```python
from build123d import *

# Parameters (mm, degrees)
SKETCH1_W           = 2
SKETCH1_H           = 6
BOSS_EXTRUDE1_DEPTH = 3


with BuildPart() as part:
    # Sketch1 → Boss-Extrude1 (new body)
    with BuildSketch(Plane(origin=(0, 0, 0), x_dir=(1, 0, 0), z_dir=(0, 1, 0))):
        Polygon((0, 6), (0, 0), (40, 0), (40, 6), (40, 19), (40, 25), (33, 25), (33, 13), (20, 13), (7, 13), (7, 25), (0, 25), (0, 19), align=None)
        with Locations((-1, 22)):
            Rectangle(SKETCH1_W, SKETCH1_H)
        with Locations((-1, 3)):
            Rectangle(SKETCH1_W, SKETCH1_H)
        with Locations((41, 3)):
            Rectangle(SKETCH1_W, SKETCH1_H)
        with Locations((41, 22)):
            Rectangle(SKETCH1_W, SKETCH1_H)
    extrude(amount=BOSS_EXTRUDE1_DEPTH)


solid = part.part
```
Can you work these out from the model? Positions are in its coordinate system, mm. A direction names the side the tool comes from. Coordinates: 2 decimals unless noted, no trailing zeros. Loops run counter-clockwise (first coordinate to the right, second up) from the corner with the lowest first, then second, coordinate; pieces in that order, holes last. Notation, with made-up numbers: M 64,36.25 L 98,36.25 A19 cw 98,65.25 Z; hole C -12.5,78.5 d4. An arc over 180 degrees is marked long. Put each result on its own line as item: value. Start each with the question number.
(1) Imagine slicing it at C-C on x = 25. List the corners of the cut face in (y, z) for me.
(2) Which directions (+Z, -Z, +X, -X, +Y, -Y) give clear straight access to the entire face, cutting with the end or side of a thin tool? Please do faces 1 (the face through (-1, 1, -19)), 2 (the face through (3, 1, -25)), 3 (the face through (40, 1, -12)), 4 (the face through (7, 1, -19)).
(3) Imagine slicing it at B-B on y = 0.7. List the corners of the cut face in (x, z) for me.
(4) Imagine slicing it at A-A on z = -15. List the corners of the cut face in (x, y) for me, and give its area (3 significant figures).
(5) We'd pull the mould along Z, two halves only. Please class faces 5 (the face through (41, 1, -6)), 6 (the face through (20, 1, -13)), 7 (the face through (42, 1, -3)): +Z half, -Z half, draft (parallel to the pull), parting line (faces both ways), or undercut.
(6) Will these pins go through, and if not, where does the flat tip stop? pin 1 Ø1 at (x, y) = (13, 2.5) entering from -Z; pin 2 Ø5 at (x, z) = (3.5, -8.5) entering from -Y; pin 3 Ø10 at (x, z) = (12.5, -19.5) entering from +Y; pin 4 Ø0.9 at (y, z) = (1.5, -11.5) entering from -X.
(7) I need wall thicknesses on probe 1 along X at (y, z) = (2.45, -20.5); probe 2 along X at (y, z) = (1.1, -18.25); probe 3 along Z at (x, y) = (11, 2.2). Which ranges of each line are inside material? Lowest first, please.
Worked answers:
1. outline: M 0,-13 L 3,-13 L 3,0 L 0,0 Z
2. face 1: -X, +Y, -Y
2. face 2: -Z, +X, -X, +Y, -Y
2. face 3: +X, +Y, -Y
2. face 4: -Z, +Y, -Y
3. outline: M -2,-25 L 7,-25 L 7,-13 L 33,-13 L 33,-25 L 42,-25 L 42,-19 L 40,-19 L 40,-6 L 42,-6 L 42,0 L -2,0 L -2,-6 L 0,-6 L 0,-19 L -2,-19 Z
4. outline: M 0,0 L 7,0 L 7,3 L 0,3 Z; M 33,0 L 40,0 L 40,3 L 33,3 Z
4. area: 42.0 mm2
5. face 5: undercut
5. face 6: -Z half
5. face 7: draft
6. pin 1: stops at z = -13
6. pin 2: stops at y = 0
6. pin 3: passes through
6. pin 4: stops at x = 0
7. probe 1: x = -2 to 7, 33 to 42
7. probe 2: x = 0 to 7, 33 to 40
7. probe 3: z = -13 to 0
